from build123d import *

# Parameters (mm, degrees)
ESQUISSE1_W        = 180
ESQUISSE1_H        = 10
BOSS_EXTRU_1_DEPTH = 0.2
ESQUISSE3_W        = 5
ESQUISSE3_H        = 5
BOSS_EXTRU_2_DEPTH = 1.5


with BuildPart() as part:
    # Esquisse1 → Boss.-Extru.1 (new body)
    with BuildSketch(Plane(origin=(0, 0, 0), x_dir=(1, 0, 0), z_dir=(0, 1, 0))):
        Rectangle(ESQUISSE1_W, ESQUISSE1_H)
    extrude(amount=BOSS_EXTRU_1_DEPTH)

    # Esquisse3 → Boss.-Extru.2 (add)
    with BuildSketch(Plane(origin=(0, 0.2, 0), x_dir=(1, 0, 0), z_dir=(0, 1, 0))):
        with Locations((45.25, 0)):
            Rectangle(ESQUISSE3_W, ESQUISSE3_H)
        with Locations((16.75, 0)):
            Rectangle(ESQUISSE3_W, ESQUISSE3_H)
        with Locations((73.75, 0)):
            Rectangle(ESQUISSE3_W, ESQUISSE3_H)
        with Locations((-73.75, 0)):
            Rectangle(ESQUISSE3_W, ESQUISSE3_H)
        with Locations((-45.25, 0)):
            Rectangle(ESQUISSE3_W, ESQUISSE3_H)
        with Locations((-16.75, 0)):
            Rectangle(ESQUISSE3_W, ESQUISSE3_H)
    extrude(amount=BOSS_EXTRU_2_DEPTH)


solid = part.part
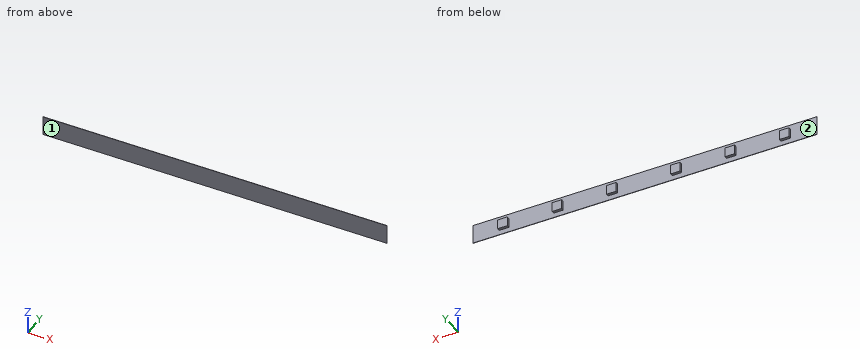
Geometry check sheet. Reference: the model listing, model coordinates, mm. Face numbers are marked on the shaded views. Give positions to 0.01 mm unless a question says otherwise; leave off trailing zeros. Loops run counter-clockwise (first coordinate to the right, second up) from the corner with the lowest first, then second, coordinate; pieces in that order, holes last. Notation, with made-up numbers: (-38.75, 68) -> (3.25, 68) arc R16 cw to (3.25, 76) -> close; hole circle Ø6 at (54.25, 41). An arc over 180 degrees is marked (long way). Answer in a Markdown table with one row per item. Add a question column.
1) Cross-section at A-A on y = 0.8. Record the boundary of the cut face in (x, z).
2) Draft check along X on the marked faces 1 and 2. Enter one of: pulls with the +X half, pulls with the -X half, needs draft (parallel to the pull), parting line crosses it, or undercut.
3) Material ranges on probe 1 along X at (y, z) = (1.05, 0.5); probe 2 along Y at (x, z) = (-14, 1); probe 3 along Z at (x, y) = (76, 1.2), recorded low to high. Write a range as from..to.
4) Cross-section at C-C on x = -46. Record the boundary of the cut face in (y, z).
5) Gauge pin test, flat ends, axial feed: P1, Ø0.8, axis at x = -45.5, y = 1, coming from the +Z side; P2, Ø6, axis at x = 9, z = -2.5, coming from the +Y side; P3, Ø0.8, axis at y = 1, z = -0.5, coming from the -X side. Record the tip position at first contact, or that the pin passes through.
6) Cross-section at B-B on z = -1. Record the boundary of the cut face in (x, y).
7) Cross-section at D-D on x = -2.5. Record the boundary of the cut face in (y, z).
Outcome:
| question | item | result |
|---|---|---|
| 1 | outline | (-76.25, -2.5) -> (-71.25, -2.5) -> (-71.25, 2.5) -> (-76.25, 2.5) -> close; (-47.75, -2.5) -> (-42.75, -2.5) -> (-42.75, 2.5) -> (-47.75, 2.5) -> close; (-19.25, -2.5) -> (-14.25, -2.5) -> (-14.25, 2.5) -> (-19.25, 2.5) -> close; (14.25, -2.5) -> (19.25, -2.5) -> (19.25, 2.5) -> (14.25, 2.5) -> close; (42.75, -2.5) -> (47.75, -2.5) -> (47.75, 2.5) -> (42.75, 2.5) -> close; (71.25, -2.5) -> (76.25, -2.5) -> (76.25, 2.5) -> (71.25, 2.5) -> close |
| 2 | face 1 | needs draft |
| 2 | face 2 | undercut |
| 3 | probe 1 | x = -76.25..-71.25, -47.75..-42.75, -19.25..-14.25, 14.25..19.25, 42.75..47.75, 71.25..76.25 |
| 3 | probe 2 | y = 0..0.2 |
| 3 | probe 3 | z = -2.5..2.5 |
| 4 | outline | (0, -5) -> (0.2, -5) -> (0.2, -2.5) -> (1.7, -2.5) -> (1.7, 2.5) -> (0.2, 2.5) -> (0.2, 5) -> (0, 5) -> close |
| 5 | P1 | stops at z = 2.5 |
| 5 | P2 | stops at y = 0.2 |
| 5 | P3 | stops at x = -76.25 |
| 6 | outline | (-90, 0) -> (90, 0) -> (90, 0.2) -> (76.25, 0.2) -> (76.25, 1.7) -> (71.25, 1.7) -> (71.25, 0.2) -> (47.75, 0.2) -> (47.75, 1.7) -> (42.75, 1.7) -> (42.75, 0.2) -> (19.25, 0.2) -> (19.25, 1.7) -> (14.25, 1.7) -> (14.25, 0.2) -> (-14.25, 0.2) -> (-14.25, 1.7) -> (-19.25, 1.7) -> (-19.25, 0.2) -> (-42.75, 0.2) -> (-42.75, 1.7) -> (-47.75, 1.7) -> (-47.75, 0.2) -> (-71.25, 0.2) -> (-71.25, 1.7) -> (-76.25, 1.7) -> (-76.25, 0.2) -> (-90, 0.2) -> close |
| 7 | outline | (0, -5) -> (0.2, -5) -> (0.2, 5) -> (0, 5) -> close |
